from build123d import *

# Parameters (mm, degrees)
SKETCH_1_W          = 20
SKETCH_1_H          = 20
SKETCH_1_W_2        = 18
SKETCH_1_H_2        = 18
EXTRUDE_1_DEPTH     = 600
SKETCH_2_R          = 1.6
CUT_EXTRUDE_1_DEPTH = 21


with BuildPart() as part:
    # 草图1 → 凸台-拉伸1 (new body)
    with BuildSketch(Plane.XY):
        Rectangle(SKETCH_1_W, SKETCH_1_H)
        Rectangle(SKETCH_1_W_2, SKETCH_1_H_2, mode=Mode.SUBTRACT)
    extrude(amount=EXTRUDE_1_DEPTH)

    # 草图2 → 切除-拉伸1 (cut, through all)
    with BuildSketch(Plane(origin=(0, 10, 0), x_dir=(1, 0, 0), z_dir=(0, 1, 0))):
        with Locations((0, -15)):
            Circle(SKETCH_2_R)
        with Locations((0, -40)):
            Circle(SKETCH_2_R)
        with Locations((0, -65)):
            Circle(SKETCH_2_R)
        with Locations((0, -90)):
            Circle(SKETCH_2_R)
        with Locations((0, -115)):
            Circle(SKETCH_2_R)
        with Locations((0, -140)):
            Circle(SKETCH_2_R)
        with Locations((0, -165)):
            Circle(SKETCH_2_R)
        with Locations((0, -190)):
            Circle(SKETCH_2_R)
        with Locations((0, -215)):
            Circle(SKETCH_2_R)
        with Locations((0, -240)):
            Circle(SKETCH_2_R)
        with Locations((0, -265)):
            Circle(SKETCH_2_R)
        with Locations((0, -290)):
            Circle(SKETCH_2_R)
        with Locations((0, -315)):
            Circle(SKETCH_2_R)
        with Locations((0, -340)):
            Circle(SKETCH_2_R)
        with Locations((0, -365)):
            Circle(SKETCH_2_R)
        with Locations((0, -390)):
            Circle(SKETCH_2_R)
        with Locations((0, -415)):
            Circle(SKETCH_2_R)
        with Locations((0, -440)):
            Circle(SKETCH_2_R)
        with Locations((0, -465)):
            Circle(SKETCH_2_R)
        with Locations((0, -490)):
            Circle(SKETCH_2_R)
        with Locations((0, -515)):
            Circle(SKETCH_2_R)
        with Locations((0, -540)):
            Circle(SKETCH_2_R)
        with Locations((0, -565)):
            Circle(SKETCH_2_R)
        with Locations((0, -590)):
            Circle(SKETCH_2_R)
    extrude(amount=-CUT_EXTRUDE_1_DEPTH, mode=Mode.SUBTRACT)


solid = part.part
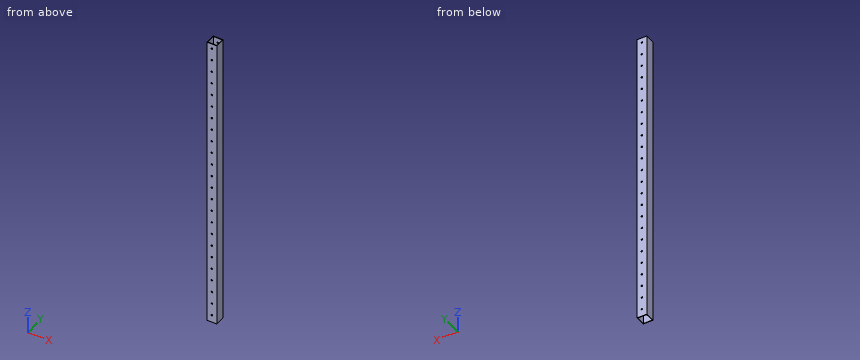
Check sheet for the modelled part. Datum: model origin and axes. Units: mm. Round coordinates to 2 decimals unless told otherwise and drop trailing zeros. Order: outer loops, then holes, each group sorted by start corner. A loop starts at its lowest first (then second) coordinate and runs counter-clockwise, first axis right, second up.
Q1. Scan lines: L1, parallel to X at y = 9.5, z = 215; L2, parallel to X at y = -7, z = 351.5. Record each from-to range of solid material in increasing order.
Filled sheet:
L1: x = -10 to -1.6, 1.6 to 10
L2: x = -10 to -9, 9 to 10
Q2. Cross-section at A-A, the plane x = -5.25. Enter the section's corners in (y, z).
Filled sheet:
outline: (-10, 0) - (-9, 0) - (-9, 600) - (-10, 600) - close; (9, 0) - (10, 0) - (10, 600) - (9, 600) - close
Q3. Cross-section at C-C, the plane z = 472. Enter the section's corners in (x, y), plus the area to 3 significant figures.
Filled sheet:
outline: (-10, -10) - (10, -10) - (10, 10) - (-10, 10) - close; hole (-9, -9) - (9, -9) - (9, 9) - (-9, 9) - close
area: 76.0 mm2
